Check sheet for the modelled part. Datum: model origin and axes. Units: mm. A direction names the side the tool comes from. Give positions to 0.01 mm unless a question says otherwise; leave off trailing zeros. Write each loop counter-clockwise with the first axis right and the second up, starting at its lowest first coordinate (ties: lowest second). Pieces come first, ordered by that corner, then holes. Notation, with made-up numbers: (86.5, 70) -> (136.5, 70) arc R31 ccw to (136.5, 100) -> close; hole circle Ø6 at (85.25, -30.75). An arc over 180 degrees is marked (long way). Use a Markdown table: item, result. Add a question column.
1. Gauge pin test, flat ends, axial feed: P1, Ø1, axis at y = -2, z = -2.5, coming from the +X side; P2, Ø2.5, axis at x = 0, y = 0, coming from the +Z side; P3, Ø1, axis at x = 1.5, z = 2.5, coming from the +Y side. Record the tip position at first contact, or that the pin passes through.
2. Set-up check for faces 1 (the flat face through (0, 0, -5.5)), 2 (the cylindrical face through (-0.54, -2.44, 0.21)), 3 (the cylindrical face through (-0.17, 1.29, 10.57)): record each of +Z, -Z, +X, -X, +Y, -Y from which the full face is reachable in a straight line by a thin tool's end or side.
3. Cross-section at C-C (z = -10). Enter the section's corners in (x, y).
4. Cross-section at D-D (z = -2.5). Enter the section's corners in (x, y), then the cut area to 3 significant figures.
5. Cross-section at A-A (x = 0). Enter the section's corners in (y, z), then the cut area to 3 significant figures.
6. Scan lines: probe 1 along Y at (x, z) = (0, 10.25); probe 2 along Y at (x, z) = (1.05, -8.5). Record each from-to range of solid material in increasing order. Write a range as [from, to].
from build123d import *

# Parameters (mm, degrees)
F0_R     = 2.5
F1_DEPTH = 15.5
F2_R     = 1.3
F3_DEPTH = 10
F4_R     = 1.3
F5_DEPTH = 10
F6_SIZE  = 0.2


with BuildPart() as f1:
    # F0 (on Top) → F1 (new body, symmetric)
    with BuildSketch(Plane.XY):
        Circle(F0_R)
    extrude(amount=F1_DEPTH, both=True)

    # F2 (on face) → F3 (cut)
    with BuildSketch(Plane.XY.offset(15.5)):
        Circle(F2_R)
    extrude(amount=-F3_DEPTH, mode=Mode.SUBTRACT)

    # F4 (on face) → F5 (cut)
    with BuildSketch(Plane(origin=(0, 0, -15.5), x_dir=(1, 0, 0), z_dir=(0, 0, -1))):
        Circle(F4_R)
    extrude(amount=-F5_DEPTH, mode=Mode.SUBTRACT)

    # F6
    f6_edges = [f1.edges().sort_by_distance(p)[0] for p in [
        (-2.5, 0, -15.5),
        (2.5, 0, 0),
        (-2.5, 0, 15.5),
    ]]
    chamfer(f6_edges, length=F6_SIZE)


solid = f1.part
Worked answers:
| question | item | result |
|---|---|---|
| 1 | P1 | stops at x = 2 |
| 1 | P2 | stops at z = 5.5 |
| 1 | P3 | stops at y = 2.29 |
| 2 | face 1 | -Z |
| 2 | face 2 | +Z, -Z |
| 2 | face 3 | +Z |
| 3 | outline | circle Ø5 at (0, 0); hole circle Ø2.6 at (0, 0) |
| 4 | outline | circle Ø5 at (0, 0) |
| 4 | area | 19.6 mm² |
| 5 | outline | (-2.5, -15.3) -> (-2.3, -15.5) -> (-1.3, -15.5) -> (-1.3, -5.5) -> (1.3, -5.5) -> (1.3, -15.5) -> (2.3, -15.5) -> (2.5, -15.3) -> (2.5, 15.3) -> (2.3, 15.5) -> (1.3, 15.5) -> (1.3, 5.5) -> (-1.3, 5.5) -> (-1.3, 15.5) -> (-2.3, 15.5) -> (-2.5, 15.3) -> close |
| 5 | area | 103 mm² |
| 6 | probe 1 | y = [-2.5, -1.3], [1.3, 2.5] |
| 6 | probe 2 | y = [-2.27, -0.77], [0.77, 2.27] |
